Work out the finished part from the listing and answer in its coordinate system (mm). A direction names the side the tool comes from. Round coordinates to 2 decimals unless told otherwise and drop trailing zeros. Write each loop counter-clockwise with the first axis right and the second up, starting at its lowest first coordinate (ties: lowest second). Pieces come first, ordered by that corner, then holes. Notation, with made-up numbers: (-5.75, 47) -> (0.25, 47) arc R19 ccw to (0.25, 52) -> close; hole circle Ø2 at (88.5, -4.5). An arc over 180 degrees is marked (long way). One line per question, with ' | ' between items. Start each with the question number.
```python
from build123d import *

# Parameters (mm, degrees)
SKETCH1_R           = 1.55
BOSS_EXTRUDE1_DEPTH = 6.35
FILLET1_R           = 10
FILLET2_R           = 10
SKETCH2_R           = 1.55
CUT_EXTRUDE1_DEPTH  = 10


with BuildPart() as part:
    # Sketch1 → Boss-Extrude1 (new body)
    with BuildSketch(Plane.XY):
        with BuildLine():
            ThreePointArc((0, 15), (-15, 0), (0, -15))
            Line((0, -15), (49.496886927, -15))
            Line((49.496886927, -15), (83.526826454, -108.496490436))
            Line((83.526826454, -108.496490436), (111.717605078, -98.235886137))
            Line((111.717605078, -98.235886137), (70.503113073, 15))
            Line((70.503113073, 15), (0, 15))
        make_face()
        with Locations((0, -8)):
            Circle(SKETCH1_R, mode=Mode.SUBTRACT)
        with Locations((-8, 0)):
            Circle(SKETCH1_R, mode=Mode.SUBTRACT)
        Circle(SKETCH1_R, mode=Mode.SUBTRACT)
        with Locations((0, 8)):
            Circle(SKETCH1_R, mode=Mode.SUBTRACT)
        with BuildLine():
            ThreePointArc((6.45, 0), (8, 1.55), (9.55, 0))
            ThreePointArc((9.55, 0), (8, -1.55), (6.45, 0))
        make_face(mode=Mode.SUBTRACT)
    extrude(amount=BOSS_EXTRUDE1_DEPTH)

    # Fillet1
    fillet1_edges = [part.edges().sort_by_distance(p)[0] for p in [
        (49.496886927, -15, 3.175),
        (70.503113073, 15, 3.175),
    ]]
    fillet(fillet1_edges, radius=FILLET1_R)

    # Fillet2
    fillet2_edges = [part.edges().sort_by_distance(p)[0] for p in [
        (111.717605078, -98.235886137, 3.175),
        (83.526826454, -108.496490436, 3.175),
    ]]
    fillet(fillet2_edges, radius=FILLET2_R)

    # Sketch2 → Cut-Extrude1 (cut)
    with BuildSketch(Plane.XY.offset(6.35)):
        with Locations((94.202014333, -93.969262079)):
            Circle(SKETCH2_R)
        with Locations((94.202014333, -88.969262079)):
            Circle(SKETCH2_R)
    extrude(amount=-CUT_EXTRUDE1_DEPTH, mode=Mode.SUBTRACT)


solid = part.part
```
(1) The mould has two halves that part along X. Classify faces 1 (the flat face through (60, -32, 0)), 2 (the cylindrical face through (7.664, 1.513, 3.131)), 3 (the cylindrical face through (85.4, -104.8, 3.2)), 4 (the flat face through (90.845, -40.89, 3.131)): +X half, -X half, draft (parallel to the pull), parting line (faces both ways), or undercut.
(2) Consider L1, parallel to Y at x = 0, z = 5; L2, parallel to Y at x = 8, z = 2.5; L3, parallel to Y at x = 31, z = 3.5. Determine where each line is inside the solid, lowest interval first.
(3) A cutting plane is placed at D-D, the plane x = 100. Determine the outline of the cut face in (y, z), then the cut area to 3 significant figures.
(4) A cutting plane is placed at C-C, the plane y = -8. Determine the outline of the cut face in (x, z), then the cut area to 3 significant figures.
(5) A cutting plane is placed at B-B, the plane z = 4.5. Determine the outline of the cut face in (x, y).
(6) For faces 5 (the cylindrical face through (95.634, -94.563, 3.219)), 6 (the flat face through (21, -15, 3)), determine the directions among +Z, -Z, +X, -X, +Y, -Y from which every point of the face is accessible in a straight line to the end or side of a thin tool.
(7) A cutting plane is placed at A-A, the plane x = 8. Determine the outline of the cut face in (y, z).
(8) Given pin 1 Ø2 at (y, z) = (-82.5, 4.5) entering from -X; pin 2 Ø4 at (x, y) = (94.2, -93.97) entering from +Z; pin 3 Ø1.5 at (y, z) = (-33.5, 1) entering from -X; pin 4 Ø2.5 at (x, y) = (0, 8) entering from -Z, each flat-ended and moving along its own axis, determine where each tip first touches the part or whether it passes through.
Returned:
1) face 1: draft | face 2: undercut | face 3: parting line | face 4: +X half
2) L1: -15 to -9.55, -6.45 to -1.55, 1.55 to 6.45, 9.55 to 15 | L2: -15 to -1.55, 1.55 to 15 | L3: -15 to 15
3) outline: (-102.5, 0) -> (-66.04, 0) -> (-66.04, 6.35) -> (-102.5, 6.35) -> close | area: 232 mm2
4) outline: (-12.69, 0) -> (-1.55, 0) -> (-1.55, 6.35) -> (-12.69, 6.35) -> close; (1.55, 0) -> (78.87, 0) -> (78.87, 6.35) -> (1.55, 6.35) -> close | area: 562 mm2
5) outline: (0, -15) -> (42.49, -15) arc R10 cw to (51.89, -21.58) -> (80.11, -99.1) arc R10 ccw to (92.92, -105.08) -> (102.32, -101.66) arc R10 ccw to (108.3, -88.84) -> (72.9, 8.42) arc R10 ccw to (63.5, 15) -> (0, 15) arc R15 ccw to start; hole circle Ø3.1 at (-8, 0); hole circle Ø3.1 at (0, -8); hole circle Ø3.1 at (0, 0); hole circle Ø3.1 at (0, 8); hole circle Ø3.1 at (8, 0); hole circle Ø3.1 at (94.2, -93.97); hole circle Ø3.1 at (94.2, -88.97)
6) face 5: +Z, -Z | face 6: +Z, -Z, -X, -Y
7) outline: (-15, 0) -> (-1.55, 0) -> (-1.55, 6.35) -> (-15, 6.35) -> close; (1.55, 0) -> (15, 0) -> (15, 6.35) -> (1.55, 6.35) -> close
8) pin 1: x = 73.7 | pin 2: z = 6.35 | pin 3: x = 55.96 | pin 4: through
